CAD build for the part. Positions are in the model's coordinates, mm. A direction names the side the tool comes from. Coordinates: 2 decimals unless noted, no trailing zeros. Loops run counter-clockwise (first coordinate to the right, second up) from the corner with the lowest first, then second, coordinate; pieces in that order, holes last.
1) Saw through at C-C, the plane z = -15.25. Write the cut outline in (x, y) (3 decimals).
2) Which spindle directions (+Z, -Z, +X, -X, +Y, -Y) get a long thin tool onto all of the face, cutting with end or side? Do faces 4 (the cylindrical face through (1.6, 5.09, -6.87)), 5 (the flat face through (0, 0, -16.9)), 6 (the flat face through (1, 0, -11.6)). Say none if no direction does.
3) Two-plate mould, pull along Y, no slides. Class faces 1 (the flat face through (-5, 0, -11.6)), 2 (the cylindrical face through (0.272, -6.184, -1.014)), 3 (the cylindrical face through (-1.734, -2.262, -5.719)): +Y half, -Y half, draft (parallel to the pull), parting line (faces both ways), or undercut.
4) Saw through at D-D, the plane x = 1.75. Write the cut outline in (y, z).
5) Pin check, flat tips, straight feed: pin 1 Ø4.5 at (x, y) = (0, 0) entering from +Z; pin 2 Ø5 at (y, z) = (4, -14.5) entering from +X. Stop position of each tip, or through.
6) Saw through at B-B, the plane x = -2.5. Write the cut outline in (y, z).
7) Saw through at A-A, the plane z = -7.5. Write the cut outline in (x, y) (3 decimals), and give its area (3 significant figures).
8) Wall check: line 1 along X through (y, z) = (0, -5.75) (3 decimals); line 2 along X through (y, z) = (0, -1.5) (3 decimals); line 3 along Z through (x, y) = (5.75, 1.25). Give the ranges that are in metal, low to high.
```python
from build123d import *


with BuildPart() as part:
    # Sketch1 → Revolve1 (revolve)
    with BuildSketch(Plane(origin=(0, 0, 0), x_dir=(0, 0, -1), z_dir=(1, 0, 0))):
        with BuildLine():
            Line((0, 2.85), (0, 6.19))
            Line((0, 6.19), (2, 6.19))
            Line((2, 6.19), (2, 5.335))
            Line((2, 5.335), (11.6, 5.335))
            Line((11.6, 5.335), (11.6, 4.725))
            Line((11.6, 4.725), (16.9, 4.725))
            Line((16.9, 4.725), (16.9, 0))
            Line((16.9, 0), (1.046838235, 0))
            Line((1.046838235, 0), (1.046838235, 0.137205882))
            ThreePointArc((1.046838235, 0.137205882), (1.193284845, 0.490759273), (1.546838235, 0.637205882))
            Line((1.546838235, 0.637205882), (11.6, 0.637205882))
            Line((11.6, 0.637205882), (11.6, 2.85))
            Line((11.6, 2.85), (0, 2.85))
        make_face()
    revolve(axis=Axis((0, 0, 5.006617647), (0, 0, -1)))


solid = part.part
```
Data:
1. outline: circle Ø9.45 at (0, 0)
2. face 4: -Z
2. face 5: -Z, +X, -X, +Y, -Y
2. face 6: +Z
3. face 1: draft
3. face 2: parting line
3. face 3: undercut
4. outline: (-5.94, -2) - (-5.04, -2) - (-5.04, -11.6) - (-4.39, -11.6) - (-4.39, -16.9) - (4.39, -16.9) - (4.39, -11.6) - (5.04, -11.6) - (5.04, -2) - (5.94, -2) - (5.94, 0) - (2.25, 0) - (2.25, -11.6) - (-2.25, -11.6) - (-2.25, 0) - (-5.94, 0) - close
5. pin 1: stops at z = -1.05
5. pin 2: stops at x = 4.48
6. outline: (-5.66, -2) - (-4.71, -2) - (-4.71, -11.6) - (-4.01, -11.6) - (-4.01, -16.9) - (4.01, -16.9) - (4.01, -11.6) - (4.71, -11.6) - (4.71, -2) - (5.66, -2) - (5.66, 0) - (1.37, 0) - (1.37, -11.6) - (-1.37, -11.6) - (-1.37, 0) - (-5.66, 0) - close
7. outline: circle Ø10.67 at (0, 0); circle Ø1.274 at (0, 0); hole circle Ø5.7 at (0, 0)
7. area: 65.2 mm2
8. line 1: x = -5.335 to -2.85, -0.637 to 0.637, 2.85 to 5.335
8. line 2: x = -6.19 to -2.85, -0.635 to 0.635, 2.85 to 6.19
8. line 3: z = -2 to 0
